Could you check a few things on this model? Use its own coordinates, in mm. A direction names the side the tool comes from. Give positions to 0.01 mm unless a question says otherwise; leave off trailing zeros. Loops run counter-clockwise (first coordinate to the right, second up) from the corner with the lowest first, then second, coordinate; pieces in that order, holes last. Notation, with made-up numbers: (52.5, 73.5) - (110.5, 73.5) arc R28 cw to (110.5, 110.5) - close; hole circle Ø9 at (60, 1). An arc over 180 degrees is marked (long way). One line per item, written item: value. Start each with the question number.
Q1. I want a section at A-A (z = -12.5). Please give me the cut outline in (x, y), then the cut area to 3 significant figures.
Q2. For faces 1 (the face through (31.22, -2.03, 22.89)), 2 (the face through (34, 14, -25)), 3 (the face through (-34, 6, 13.5)), 4 (the face through (1, 7, 28.9)), which set-ups out of +Z, -Z, +X, -X, +Y, -Y let a thin tool reach every point of the face, with its end or its side?
Q3. I want a section at C-C (y = 5.5). Please give me the cut outline in (x, z).
Q4. I want a section at B-B (x = -22.5). Please give me the cut outline in (y, z).
Q5. I want a section at D-D (z = 16). Please give me the cut outline in (x, y), then the cut area to 3 significant figures.
Q6. If I drill on line 1 (X direction, y = -1.6, z = -9.5); line 2 (Z direction, x = -18, y = -1.65); line 3 (Y direction, x = 34, z = -25), over which ranges is the centre line in solid material (lowest first)? Write a range as from..to.
Q7. If we mould it in two halves opening along X, with no side actions, what happens to faces 5 (the face through (33, -4, -9)), 6 (the face through (35.5, -0.3, 0.1)), 7 (the face through (34, 9, -19))? For each: released by +X, released by -X, zero draft, split by the parting line, or undercut.
Q8. I'm going to push flat-ended pins straight in: P1, Ø12, axis at y = 11.5, z = 6, coming from the +X side; P2, Ø10, axis at x = 15.5, z = -1.5, coming from the +Y side; P3, Ø2.5, axis at x = -16.5, z = 25, coming from the -Y side; P4, Ø0.8, axis at x = 4, y = -5, coming from the +Z side. Where does each tip first touch, or does it pass through?
```python
from build123d import *

# Parameters (mm, degrees)
EXTRUDE_1_DEPTH      = 4
SKETCH_3_W           = 73
SKETCH_3_H           = 58
EXTRUDE_2_DEPTH      = 13
EXTRUDE_2_DEPTH_BACK = 4
SKETCH_4_W           = 17
SKETCH_4_H           = 7
EXTRUDE_4_DEPTH      = 4
SKETCH_5_R           = 1.5
CUT_EXTRUDE_1_DEPTH  = 4
EXTRUDE_5_DEPTH      = 4
EXTRUDE_6_DEPTH      = 4
SKETCH_8_W           = 73
SKETCH_8_H           = 58
EXTRUDE_7_DEPTH      = 1
SKETCH_9_W           = 8.5
SKETCH_9_H           = 3.5
CUT_EXTRUDE_2_DEPTH  = 2
CHAMFER_1_SIZE       = 0.5
SKETCH_10_W          = 9
SKETCH_10_H          = 12
CUT_EXTRUDE_3_DEPTH  = 2
CHAMFER_2_SIZE       = 0.5
CHAMFER_3_SIZE       = 0.5
CHAMFER_4_SIZE       = 0.5
CUT_EXTRUDE_4_DEPTH  = 2
CHAMFER_5_SIZE       = 0.5
CHAMFER_6_SIZE       = 0.5
SKETCH_21_W          = 2
SKETCH_21_H          = 58
CUT_EXTRUDE_5_DEPTH  = 19
CUT_EXTRUDE_7_DEPTH  = 13
EXTRUDE_8_DEPTH      = 6
SKETCH_36_W          = 71
SKETCH_36_H          = 39.5
EXTRUDE_9_DEPTH      = 1.5
SKETCH_39_R          = 1
CUT_EXTRUDE_9_DEPTH  = 5
SKETCH_42_W          = 9.25
SKETCH_42_H          = 0.2
CUT_EXTRUDE_10_DEPTH = 72
SKETCH_43_W          = 0.1
SKETCH_43_H          = 23.8
CUT_EXTRUDE_11_DEPTH = 72
CUT_EXTRUDE_12_DEPTH = 0.5
CUT_EXTRUDE_13_DEPTH = 0.5
SKETCH_46_W          = 66.5
SKETCH_46_H          = 54.4
SKETCH_46_W_2        = 66
SKETCH_46_H_2        = 54
CUT_EXTRUDE_14_DEPTH = 19
SKETCH_47_W          = 11.5
SKETCH_47_H          = 6.5
SKETCH_47_W_2        = 8.5
SKETCH_47_H_2        = 3.5
CUT_EXTRUDE_16_DEPTH = 7.5
CUT_EXTRUDE_17_DEPTH = 7.5
SKETCH_51_W          = 10
SKETCH_51_H          = 14.5
SKETCH_51_W_2        = 7.5
SKETCH_51_H_2        = 12
CUT_EXTRUDE_18_DEPTH = 7.5


with BuildPart() as part:
    # 草图1 → 凸台-拉伸1 (new body)
    with BuildSketch(Plane(origin=(0, 0, 0), x_dir=(1, 0, 0), z_dir=(0, 1, 0))):
        Polygon((33, -27), (-33, -27), (-33, 27), (33, 27), (33, 14), (36, 11), (36, -21), (33, -24), align=None)
        Polygon((-31.777777778, 26), (-31.777777778, -26), (31.777777778, -26), (31.777777778, -23.80800866), (35, -20.585786438), (35, 9.543812347), (35, 10.585786438), (31.777777778, 13.80800866), (31.777777778, 26), align=None, mode=Mode.SUBTRACT)
    extrude(amount=-EXTRUDE_1_DEPTH)

    # 草图3 → 凸台-拉伸2 (add, two sides)
    with BuildSketch(Plane(origin=(0, 0, 0), x_dir=(1, 0, 0), z_dir=(0, 1, 0))) as extrude_2_sk:
        with Locations((1.5, 0)):
            Rectangle(SKETCH_3_W, SKETCH_3_H)
        Polygon((33, 27), (33, 14), (36, 11), (36, -21), (33, -24), (33, -27), (-33, -27), (-33, 27), align=None, mode=Mode.SUBTRACT)
    extrude(amount=EXTRUDE_2_DEPTH)
    extrude(extrude_2_sk.sketch, amount=-EXTRUDE_2_DEPTH_BACK)

    # 草图4 → 凸台-拉伸4 (add)
    with BuildSketch(Plane(origin=(0, 0, 0), x_dir=(1, 0, 0), z_dir=(0, 1, 0))):
        with Locations((-23.277777778, 22.5)):
            Rectangle(SKETCH_4_W, SKETCH_4_H)
        Polygon((31.777777778, 13.80800866), (27.777777778, 13.80800866), (27.777777778, -22), (33.585786438, -22), (35, -20.585786438), (35, 10.585786438), align=None)
    extrude(amount=-EXTRUDE_4_DEPTH)

    # 草图5 → 切除-拉伸1 (cut)
    with BuildSketch(Plane(origin=(0, 0, 0), x_dir=(1, 0, 0), z_dir=(0, 1, 0))):
        with Locations((-18, 25)):
            Circle(SKETCH_5_R)
        with Locations((33.5, 9.5)):
            Circle(SKETCH_5_R)
        with Locations((33.5, -18.5)):
            Circle(SKETCH_5_R)
    extrude(amount=-CUT_EXTRUDE_1_DEPTH, mode=Mode.SUBTRACT)

    # 草图6 → 凸台-拉伸5 (add)
    with BuildSketch(Plane.XZ.offset(4)):
        Polygon((31.777777778, 23.80800866), (33.585786438, 22), (30.681782108, 22), align=None)
    extrude(amount=-EXTRUDE_5_DEPTH)

    # 草图7 → 凸台-拉伸6 (add)
    with BuildSketch(Plane(origin=(0, 0, 0), x_dir=(1, 0, 0), z_dir=(0, 1, 0))):
        Polygon((-14.158955627, 26), (-14.777777778, 19), (-14.777777778, 26), align=None)
    extrude(amount=-EXTRUDE_6_DEPTH)

    # 草图8 → 凸台-拉伸7 (add)
    with BuildSketch(Plane.XZ.offset(4)):
        with Locations((1.5, 0)):
            Rectangle(SKETCH_8_W, SKETCH_8_H)
    extrude(amount=EXTRUDE_7_DEPTH)

    # 草图9 → 切除-拉伸2 (cut)
    with BuildSketch(Plane(origin=(-33, 0, 0), x_dir=(0, 0, -1), z_dir=(1, 0, 0))):
        with Locations((10.25, 2.75)):
            Rectangle(SKETCH_9_W, SKETCH_9_H)
    extrude(amount=-CUT_EXTRUDE_2_DEPTH, mode=Mode.SUBTRACT)

    # 倒角1
    chamfer_1_edges = [part.edges().sort_by_distance(p)[0] for p in [
        (-35, 4.5, -10.25),
        (-35, 2.75, -14.5),
        (-35, 1, -10.25),
        (-35, 2.75, -6),
    ]]
    chamfer(chamfer_1_edges, length=CHAMFER_1_SIZE)

    # 草图10 → 切除-拉伸3 (cut)
    with BuildSketch(Plane(origin=(-33, 0, 0), x_dir=(0, 0, -1), z_dir=(1, 0, 0))):
        with Locations((-18.5, 6)):
            Rectangle(SKETCH_10_W, SKETCH_10_H)
    extrude(amount=-CUT_EXTRUDE_3_DEPTH, mode=Mode.SUBTRACT)

    # 倒角2
    chamfer_2_edges = [part.edges().sort_by_distance(p)[0] for p in [
        (-35, 6, 23),
        (-35, 12, 18.5),
        (-35, 6, 14),
        (-35, 0, 18.5),
    ]]
    chamfer(chamfer_2_edges, length=CHAMFER_2_SIZE)

    # 倒角3
    chamfer_3_edges = [part.edges().sort_by_distance(p)[0] for p in [
        (-33, 4.5, -10.25),
        (-33, 1, -10.25),
        (-33, 12, 18.5),
    ]]
    chamfer(chamfer_3_edges, length=CHAMFER_3_SIZE)

    # 倒角4
    chamfer_4_edges = [part.edges().sort_by_distance(p)[0] for p in [
        (-33, 6, 14),
        (-33, 6, 23),
        (-33, 2.75, -6),
        (-33, 2.75, -14.5),
    ]]
    chamfer(chamfer_4_edges, length=CHAMFER_4_SIZE)

    # 草图13 → 切除-拉伸4 (cut)
    with BuildSketch(Plane(origin=(-33, 0, 0), x_dir=(0, 0, -1), z_dir=(1, 0, 0))):
        with BuildLine():
            Line((-6, 8.6), (-7.1, 8.6))
            ThreePointArc((-7.1, 8.6), (-9.4, 6.3), (-7.1, 4))
            Line((-7.1, 4), (-6, 4))
            Line((-6, 4), (-6, 8.6))
        make_face()
    extrude(amount=-CUT_EXTRUDE_4_DEPTH, mode=Mode.SUBTRACT)

    # 倒角5
    chamfer_5_edges = [part.edges().sort_by_distance(p)[0] for p in [
        (-35, 6.3, 6),
        (-35, 4, 6.55),
        (-35, 6.3, 9.4),
        (-35, 8.6, 6.55),
    ]]
    chamfer(chamfer_5_edges, length=CHAMFER_5_SIZE)

    # 倒角6
    chamfer_6_edges = [part.edges().sort_by_distance(p)[0] for p in [
        (-33, 6.3, 6),
        (-33, 8.6, 6.55),
        (-33, 6.3, 9.4),
        (-33, 4, 6.55),
    ]]
    chamfer(chamfer_6_edges, length=CHAMFER_6_SIZE)

    # 草图21 → 切除-拉伸5 (cut, through all)
    with BuildSketch(Plane(origin=(0, 13, 0), x_dir=(1, 0, 0), z_dir=(0, 1, 0))):
        with Locations((37, 0)):
            Rectangle(SKETCH_21_W, SKETCH_21_H)
    extrude(amount=-CUT_EXTRUDE_5_DEPTH, mode=Mode.SUBTRACT)

    # 草图23 → 切除-拉伸7 (cut)
    with BuildSketch(Plane(origin=(0, 13, 0), x_dir=(1, 0, 0), z_dir=(0, 1, 0))):
        Polygon((33, 14), (33, 19), (36, 19), (36, 11), align=None)
    extrude(amount=-CUT_EXTRUDE_7_DEPTH, mode=Mode.SUBTRACT)

    # 草图27 → 凸台-拉伸8 (add)
    with BuildSketch(Plane(origin=(0, 13, 0), x_dir=(1, 0, 0), z_dir=(0, 1, 0))):
        Polygon((33, 19), (36, 19), (36, 29), (-35, 29), (-35, -29), (36, -29), (36, -21), (33, -24), (33, -27), (-33, -27), (-33, 27), (33, 27), align=None)
    extrude(amount=EXTRUDE_8_DEPTH)

    # 草图36 → 凸台-拉伸9 (add)
    with BuildSketch(Plane.XZ.offset(5)):
        with Locations((0.5, 0)):
            Rectangle(SKETCH_36_W, SKETCH_36_H)
    extrude(amount=EXTRUDE_9_DEPTH)

    # 草图39 → 切除-拉伸9 (cut)
    with BuildSketch(Plane(origin=(36, 0, 0), x_dir=(0, 0, -1), z_dir=(1, 0, 0))):
        with Locations((-25, 15)):
            Circle(SKETCH_39_R)
        with Locations((25, 15)):
            Circle(SKETCH_39_R)
    extrude(amount=-CUT_EXTRUDE_9_DEPTH, mode=Mode.SUBTRACT)

    # 草图42 → 切除-拉伸10 (cut, through all)
    with BuildSketch(Plane(origin=(36, 0, 0), x_dir=(0, 0, -1), z_dir=(1, 0, 0))):
        with Locations((-24.375, -4.9)):
            Rectangle(SKETCH_42_W, SKETCH_42_H)
        with Locations((24.375, -4.9)):
            Rectangle(SKETCH_42_W, SKETCH_42_H)
    extrude(amount=-CUT_EXTRUDE_10_DEPTH, mode=Mode.SUBTRACT)

    # 草图43 → 切除-拉伸11 (cut, through all)
    with BuildSketch(Plane(origin=(36, 0, 0), x_dir=(0, 0, -1), z_dir=(1, 0, 0))):
        with Locations((-28.95, 7.1)):
            Rectangle(SKETCH_43_W, SKETCH_43_H)
        with Locations((28.95, 7.1)):
            Rectangle(SKETCH_43_W, SKETCH_43_H)
    extrude(amount=-CUT_EXTRUDE_11_DEPTH, mode=Mode.SUBTRACT)

    # 草图44 → 切除-拉伸12 (cut)
    with BuildSketch(Plane(origin=(36, 0, 0), x_dir=(0, 0, -1), z_dir=(1, 0, 0))):
        Polygon((19.75, -4.8), (28.9, -4.8), (28.9, 19), (19, 19), (19, 0), (-21, 0), (-21, 19), (-28.9, 19), (-28.9, -4.8), (-19.75, -4.8), (-19.75, -6.5), (19.75, -6.5), align=None)
    extrude(amount=-CUT_EXTRUDE_12_DEPTH, mode=Mode.SUBTRACT)

    # 草图45 → 切除-拉伸13 (cut)
    with BuildSketch(Plane.ZY.offset(35)):
        Polygon((28.9, 19), (-28.9, 19), (-28.9, -4.8), (-19.75, -4.8), (-19.75, -6.5), (19.75, -6.5), (19.75, -4.8), (28.9, -4.8), align=None)
    extrude(amount=-CUT_EXTRUDE_13_DEPTH, mode=Mode.SUBTRACT)

    # 草图46 → 切除-拉伸14 (cut)
    with BuildSketch(Plane(origin=(0, 19, 0), x_dir=(1, 0, 0), z_dir=(0, 1, 0))):
        with Locations((0.15, 0)):
            Rectangle(SKETCH_46_W, SKETCH_46_H)
        Rectangle(SKETCH_46_W_2, SKETCH_46_H_2, mode=Mode.SUBTRACT)
    extrude(amount=-CUT_EXTRUDE_14_DEPTH, mode=Mode.SUBTRACT)

    # 草图47 → 切除-拉伸16 (cut)
    with BuildSketch(Plane.ZY.offset(34.5)):
        with Locations((-10.75, 3.25)):
            Rectangle(SKETCH_47_W, SKETCH_47_H)
        with Locations((-10.25, 2.75)):
            Rectangle(SKETCH_47_W_2, SKETCH_47_H_2, mode=Mode.SUBTRACT)
    extrude(amount=-CUT_EXTRUDE_16_DEPTH, mode=Mode.SUBTRACT)

    # 草图48 → 切除-拉伸17 (cut)
    with BuildSketch(Plane(origin=(-33.1, 0, 0), x_dir=(0, 0, -1), z_dir=(1, 0, 0))):
        with BuildLine():
            Line((-7.1, 10), (-5.6, 10))
            Line((-5.6, 10), (-4.6, 10))
            Line((-4.6, 10), (-4.6, 2.6))
            Line((-4.6, 2.6), (-5.6, 2.6))
            Line((-5.6, 2.6), (-7.1, 2.6))
            ThreePointArc((-7.1, 2.6), (-10.8, 6.3), (-7.1, 10))
        make_face()
    extrude(amount=-CUT_EXTRUDE_17_DEPTH, mode=Mode.SUBTRACT)

    # 草图51 → 切除-拉伸18 (cut)
    with BuildSketch(Plane.ZY.offset(34.5)):
        with Locations((18.5, 5.75)):
            Rectangle(SKETCH_51_W, SKETCH_51_H)
        with Locations((17.75, 6)):
            Rectangle(SKETCH_51_W_2, SKETCH_51_H_2, mode=Mode.SUBTRACT)
    extrude(amount=-CUT_EXTRUDE_18_DEPTH, mode=Mode.SUBTRACT)


solid = part.part
```
Worked answers:
1. outline: (-34.5, -6.5) - (35.5, -6.5) - (35.5, 0) - (27.78, 0) - (27.78, -4) - (-31.78, -4) - (-31.78, 0) - (-34.5, 0) - close; (-34.5, 6.5) - (-33.1, 6.5) - (-33.1, 19) - (-34.5, 19) - close
1. area: 234 mm²
2. face 1: +Y
2. face 2: +X
2. face 3: -X
2. face 4: +Z, +X, -X, +Y, -Y
3. outline: (-34.5, -28.9) - (35.5, -28.9) - (35.5, -19) - (33.4, -19) - (33.4, -27.2) - (-33.1, -27.2) - (-33.1, -16.5) - (-34.5, -16.5) - close; (-34.5, -5) - (-33.1, -5) - (-33.1, 4.6) - (-34.5, 4.6) - close; (-34.5, 10.71) - (-33.1, 10.71) - (-33.1, 13.5) - (-34.5, 13.5) - close; (-34.5, 23.5) - (-33.1, 23.5) - (-33.1, 27.2) - (33.4, 27.2) - (33.4, 23.6) - (35.5, 21.5) - (35.5, 28.9) - (-34.5, 28.9) - close
4. outline: (-6.5, -19.75) - (-4.8, -19.75) - (-4.8, -28.9) - (19, -28.9) - (19, -27.2) - (0, -27.2) - (0, -19) - (-4, -19) - (-4, 26) - (0, 26) - (0, 27.2) - (19, 27.2) - (19, 28.9) - (-4.8, 28.9) - (-4.8, 19.75) - (-6.5, 19.75) - close
5. outline: (-34.5, -6.5) - (35.5, -6.5) - (35.5, 0) - (27.78, 0) - (27.78, -4) - (-31.78, -4) - (-31.78, -1.5) - (-34.5, -1.5) - close; (-34.5, 13) - (-33.1, 13) - (-33.1, 19) - (-34.5, 19) - close
5. area: 221 mm²
6. line 1: x = -34.5..-31.78, 27.78..32, 35..35.5
6. line 2: z = -28.9..-26.5, -23.5..-19, 26..28.9
6. line 3: y = -4.8..14, 16..19
7. face 5: undercut
7. face 6: released by +X
7. face 7: zero draft
8. P1: stops at x = -33.1
8. P2: stops at y = -4
8. P3: stops at y = -4.8
8. P4: stops at z = 28.9
